The model under review builds one solid part; all positions refer to its coordinate system, in mm. Face numbers are marked on the shaded views. A direction names the side the tool comes from. Give positions to 0.01 mm unless a question says otherwise; leave off trailing zeros. One line per question, with ' | ' between items. Start each with the question number.
```python
from build123d import *

# Parameters (mm, degrees)
SKETCH1_R             = 4
SKETCH1_R_2           = 1.5
BOSS_EXTRUDE1_DEPTH   = 10
FILLET1_R             = 3
FILLET2_R             = 1
CUT_EXTRUDE1_DEPTH    = 24
CIRPATTERN1_OUTLINE_R = 1.5
CIRPATTERN1_DEPTH     = 45
SKETCH3_W             = 15
SKETCH3_H             = 45
SKETCH3_R             = 1.5
BOSS_EXTRUDE2_DEPTH   = 10
FILLET3_R             = 5
SKETCH4_R             = 3.25
CUT_EXTRUDE2_DEPTH    = 3
SKETCH5_W             = 8
SKETCH5_H             = 8
BOSS_EXTRUDE3_DEPTH   = 1.75


# Read off the part's stored shape, not the designer's step: CirPattern1
with BuildPart() as part:
    # Sketch1 → Boss-Extrude1 (new body)
    with BuildSketch(Plane(origin=(0, 0, 0), x_dir=(1, 0, 0), z_dir=(0, 1, 0))):
        Polygon((0, 0), (-42, 0), (-42, -8), (-50, -8), (-50, -37), (-42, -37), (-42, -45), (0, -45), align=None)
        with Locations(Location((-22.5, -22.5, 0), (0, 0, 270))):
            Circle(SKETCH1_R, mode=Mode.SUBTRACT)
        with BuildLine():
            Line((-19.75, -13), (-25.25, -13))
            ThreePointArc((-25.25, -13), (-26.103553391, -13.353553391), (-25.75, -12.5))
            Line((-25.75, -12.5), (-25.75, -10))
            ThreePointArc((-25.75, -10), (-26.103553391, -9.146446609), (-25.25, -9.5))
            Line((-25.25, -9.5), (-19.75, -9.5))
            ThreePointArc((-19.75, -9.5), (-18.896446609, -9.146446609), (-19.25, -10))
            Line((-19.25, -10), (-19.25, -12.5))
            ThreePointArc((-19.25, -12.5), (-18.896446609, -13.353553391), (-19.75, -13))
        make_face(mode=Mode.SUBTRACT)
        with Locations(Location((-31.25, -8.75, 0), (0, 0, 270))):
            Circle(SKETCH1_R_2, mode=Mode.SUBTRACT)
        with Locations(Location((-31.25, -36.25, 0), (0, 0, 270))):
            Circle(SKETCH1_R_2, mode=Mode.SUBTRACT)
        with Locations(Location((-8.75, -36.25, 0), (0, 0, 270))):
            Circle(SKETCH1_R_2, mode=Mode.SUBTRACT)
        with Locations(Location((-8.75, -8.75, 0), (0, 0, 270))):
            Circle(SKETCH1_R_2, mode=Mode.SUBTRACT)
        with BuildLine():
            Line((-9.5, -19.75), (-9.5, -25.25))
            ThreePointArc((-9.5, -25.25), (-9.146446609, -26.103553391), (-10, -25.75))
            Line((-10, -25.75), (-12.5, -25.75))
            ThreePointArc((-12.5, -25.75), (-13.353553391, -26.103553391), (-13, -25.25))
            Line((-13, -25.25), (-13, -19.75))
            ThreePointArc((-13, -19.75), (-13.353553391, -18.896446609), (-12.5, -19.25))
            Line((-12.5, -19.25), (-10, -19.25))
            ThreePointArc((-10, -19.25), (-9.146446609, -18.896446609), (-9.5, -19.75))
        make_face(mode=Mode.SUBTRACT)
        with BuildLine():
            ThreePointArc((-19.25, -35), (-18.896446609, -35.853553391), (-19.75, -35.5))
            Line((-19.75, -35.5), (-25.25, -35.5))
            ThreePointArc((-25.25, -35.5), (-26.103553391, -35.853553391), (-25.75, -35))
            Line((-25.75, -35), (-25.75, -32.5))
            ThreePointArc((-25.75, -32.5), (-26.103553391, -31.646446609), (-25.25, -32))
            Line((-25.25, -32), (-19.75, -32))
            ThreePointArc((-19.75, -32), (-18.896446609, -31.646446609), (-19.25, -32.5))
            Line((-19.25, -32.5), (-19.25, -35))
        make_face(mode=Mode.SUBTRACT)
    extrude(amount=BOSS_EXTRUDE1_DEPTH)

    # Fillet1
    fillet1_edges = [part.edges().sort_by_distance(p)[0] for p in [
        (0, 5, 45),
        (0, 5, 0),
    ]]
    fillet(fillet1_edges, radius=FILLET1_R)

    # Fillet2
    fillet2_edges = [part.edges().sort_by_distance(p)[0] for p in [
        (-25.75, 5, 32.5),
        (-25.75, 5, 35),
        (-25.25, 5, 35.5),
        (-19.75, 5, 35.5),
        (-19.25, 5, 35),
        (-19.25, 5, 32.5),
        (-19.75, 5, 32),
        (-25.25, 5, 32),
        (-19.25, 5, 12.5),
        (-19.25, 5, 10),
        (-19.75, 5, 9.5),
        (-25.25, 5, 9.5),
        (-25.75, 5, 10),
        (-25.75, 5, 12.5),
        (-25.25, 5, 13),
        (-19.75, 5, 13),
        (-10, 5, 19.25),
        (-12.5, 5, 19.25),
        (-13, 5, 19.75),
        (-13, 5, 25.25),
        (-12.5, 5, 25.75),
        (-10, 5, 25.75),
        (-9.5, 5, 25.25),
    ]]
    fillet(fillet2_edges, radius=FILLET2_R)

    # Sketch2 → Cut-Extrude1 (cut)
    with BuildSketch(Plane(origin=(0, 0, 0), x_dir=(0, 0, -1), z_dir=(1, 0, 0))):
        with BuildLine():
            ThreePointArc((-21, 5), (-21.439339828, 6.060660172), (-22.5, 6.5))
            Line((-22.5, 6.5), (-22.5, 3.5))
            ThreePointArc((-22.5, 3.5), (-21.439339828, 3.939339828), (-21, 5))
        make_face()
        with BuildLine():
            Line((-22.5, 3.5), (-22.5, 6.5))
            ThreePointArc((-22.5, 6.5), (-24, 5), (-22.5, 3.5))
        make_face()
    extrude(amount=-CUT_EXTRUDE1_DEPTH, mode=Mode.SUBTRACT)

    # CirPattern1 outline → CirPattern1 (cut)
    with BuildSketch(Plane.XY):
        with Locations((-22.5, 5)):
            Circle(CIRPATTERN1_OUTLINE_R)
    extrude(amount=CIRPATTERN1_DEPTH, mode=Mode.SUBTRACT)

    # Sketch3 → Boss-Extrude2 (add)
    with BuildSketch(Plane(origin=(0, 10, 0), x_dir=(1, 0, 0), z_dir=(0, 1, 0))):
        with Locations((-57.5, -22.5)):
            Rectangle(SKETCH3_W, SKETCH3_H)
        with Locations(Location((-60, -37.5, 0), (0, 0, 270))):
            Circle(SKETCH3_R, mode=Mode.SUBTRACT)
        with Locations(Location((-60, -7.5, 0), (0, 0, 270))):
            Circle(SKETCH3_R, mode=Mode.SUBTRACT)
    extrude(amount=-BOSS_EXTRUDE2_DEPTH)

    # Fillet3
    fillet3_edges = [part.edges().sort_by_distance(p)[0] for p in [
        (-65, 5, 0),
        (-65, 5, 45),
    ]]
    fillet(fillet3_edges, radius=FILLET3_R)

    # Sketch4 → Cut-Extrude2 (cut)
    with BuildSketch(Plane.XZ):
        with Locations(Location((-31.25, 36.25, 0), (0, 0, 270))):
            Circle(SKETCH4_R)
        with Locations(Location((-8.75, 36.25, 0), (0, 0, 270))):
            Circle(SKETCH4_R)
        with Locations(Location((-8.75, 8.75, 0), (0, 0, 270))):
            Circle(SKETCH4_R)
        with Locations(Location((-31.25, 8.75, 0), (0, 0, 270))):
            Circle(SKETCH4_R)
        with Locations(Location((-60, 37.5, 0), (0, 0, 270))):
            Circle(SKETCH4_R)
        with Locations(Location((-60, 7.5, 0), (0, 0, 270))):
            Circle(SKETCH4_R)
    extrude(amount=-CUT_EXTRUDE2_DEPTH, mode=Mode.SUBTRACT)

    # Sketch5 → Boss-Extrude3 (add)
    with BuildSketch(Plane.XZ):
        with Locations((-46, 41)):
            Rectangle(SKETCH5_W, SKETCH5_H)
        with Locations((-46, 4)):
            Rectangle(SKETCH5_W, SKETCH5_H)
    extrude(amount=-BOSS_EXTRUDE3_DEPTH)


solid = part.part
```
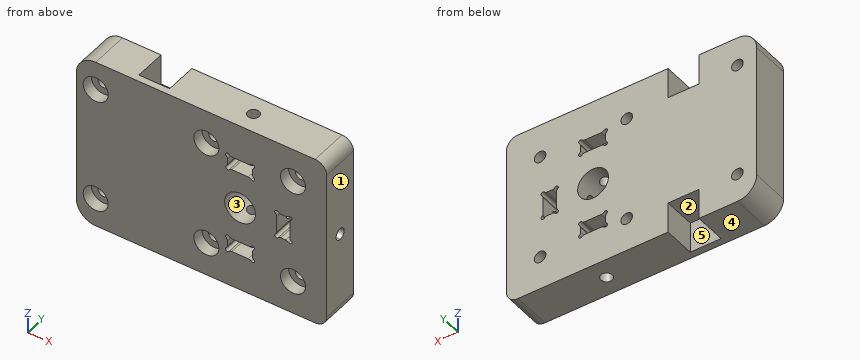
Item 1: Clearance check with flat-ended pins moving along their axes: P1, Ø4, axis at x = -45.5, z = 3.5, coming from the +Y side; P2, Ø2.5, axis at x = -31.25, z = 8.75, coming from the +Y side (3 decimals); P3, Ø4, axis at x = -46, y = 7.5, coming from the +Z side. State where each tip first meets the part, or that it passes through.
Item 2: For probe 1 along Z at (x, y) = (-22.5, 2.5); probe 2 along Z at (x, y) = (-31.25, 5.5); probe 3 along X at (y, z) = (6.25, 10), list the stretches that pass through material, from the lowest coordinate up.
Item 3: Machinability: for the marked faces 4 and 5, which of the approach directions +Z, -Z, +X, -X, +Y, -Y give a long, thin tool a straight path to every point of the face, cutting with its end or side? Answer none if there is none.
Item 4: Take a section at A-A (x = -22.5). State how many separate pieces and enclosed holes the cut face has, plus the area to 3 significant figures.
Item 5: The part is to be moulded in two halves that separate along Z. For the marked faces 1, 2 and 3, say which applies: +Z half, -Z half, draft (parallel to the pull), parting line (faces both ways), or undercut.
Check sheet entries:
1) P1: stops at y = 1.75 | P2: passes through | P3: stops at z = 37
2) probe 1: z = 0 to 9.5, 13 to 18.5, 26.5 to 32, 35.5 to 45 | probe 2: z = 0 to 7.25, 10.25 to 34.75, 37.75 to 45 | probe 3: x = -65 to -32.08, -30.42 to -25.96, -19.04 to -9.58, -7.92 to 0
3) face 4: -Z, +X, -X, +Y, -Y | face 5: -Z, +Y
4) separate pieces: 8 | enclosed holes: 0 | area: 210 mm^2
5) face 1: draft | face 2: -Z half | face 3: undercut
